from build123d import *

# Parameters (mm, degrees)
SKETCH2_R           = 46.875
BOSS_EXTRUDE1_DEPTH = 3


with BuildPart() as part:
    # Sketch1 → Revolve1 (revolve)
    with BuildSketch(Plane.XY, mode=Mode.PRIVATE) as revolve1_sk:
        Polygon((-48.883652299488276, 0), (-156.25, 61.6327346895418), (-155.75215375739506, 62.5), (-46.875, 0), align=None)
    revolve(revolve1_sk.sketch.rotate(Axis((0, 0, 0), (0, 1, 0)), 90), axis=Axis((0, 0, 0), (0, 1, 0)))



with BuildPart() as body_2:
    # Sketch2 → Boss-Extrude1 (new body)
    with BuildSketch(Plane(origin=(0, 0, 0), x_dir=(1, 0, 0), z_dir=(0, 1, 0))):
        Polygon((-156.24999999999994, -156.25), (156.25000000000003, -156.25), (156.25, 155.75215375739506), (-156.24999999999994, 155.75215375739506), align=None)
        with Locations(Location((8.327e-14, -0.24892312130248007, 0), (0, 0, 270))):
            Circle(SKETCH2_R, mode=Mode.SUBTRACT)
    extrude(amount=-BOSS_EXTRUDE1_DEPTH)


with BuildPart() as part_1:
    add(part.part)

    add(body_2.part)  # Revolve2 merges body 2
    # Sketch3 → Revolve2 (revolve)
    with BuildSketch(Plane.XY, mode=Mode.PRIVATE) as revolve2_sk:
        with BuildLine():
            Line((-65.84427513417332, 9.73610064724726), (-48.88365229948828, 0))
            Line((-48.88365229948828, 0), (-68.44009325263127, 0))
            ThreePointArc((-68.44009325263127, 0), (-63.40199024858691, 3.8708478952321843), (-65.84427513417332, 9.73610064724726))
        make_face()
    revolve(revolve2_sk.sketch.rotate(Axis((0, 0, 0), (0, 1, 0)), 270), axis=Axis((0, 0, 0), (0, 1, 0)))


solid = part_1.part
Check sheet for the modelled part. Datum: model origin and axes. Units: mm. Coordinates: 2 decimals unless noted, no trailing zeros. Loops run counter-clockwise (first coordinate to the right, second up) from the corner with the lowest first, then second, coordinate; pieces in that order, holes last. Notation, with made-up numbers: (2.25, 6) -> (16.25, 6) arc R26 ccw to (16.25, 42) -> close; hole circle Ø9 at (0, 56.25). An arc over 180 degrees is marked (long way). Write item = value, one per line. Start each with the question number.
1. Section check B-B on y = 48. Record the cut outline in (x, z).
2. Draft check along Y on faces 1 (the flat face through (-37, -3, -37)), 2 (the conical face through (-69.799, 12.983, -15.5)), 3 (the conical face through (-50.921, 3.035, -11.308)). Enter one of: released by +Y, released by -Y, zero draft, split by the parting line, or undercut.
3. Section check A-A on x = 0. Record the cut outline in (y, z) (3 decimals), then the cut area to 3 significant figures.
4. Material ranges on line 1 (Y direction, x = 106, z = -136.5); line 2 (X direction, y = 51, z = 21); line 3 (Y direction, x = -6, z = 116), recorded low to high.
5. Depth check by flat-ended pin: P1, Ø2, axis at x = 5, y = 9, coming from the +Z side; P2, Ø5, axis at y = 12, z = -43.5, coming from the -X side; P3, Ø8, axis at y = 23.5, z = -54, coming from the -X side. Enter the tip coordinate at first touch or a pass-through.
Responses:
q1.outline = circle Ø265 at (0, 0); hole circle Ø260.99 at (0, 0)
q2.face_1 = released by -Y
q2.face_2 = undercut
q2.face_3 = released by +Y
q3.outline = (-3, -155.752) -> (0, -155.752) -> (0, -68.44) arc R5.214 cw to (9.736, -65.844) -> (61.633, -156.25) -> (62.5, -155.752) -> (0, -46.875) -> (0, -46.626) -> (-3, -46.626) -> close; (-3, 47.124) -> (0, 47.124) -> (0, 46.875) -> (62.5, 155.752) -> (61.633, 156.25) -> (9.736, 65.844) arc R5.214 cw to (0, 68.44) -> (0, 156.25) -> (-3, 156.25) -> close
q3.area = 1,040 mm2
q4.line_1 = -3 to 0
q4.line_2 = -136.12 to -134.08, 134.08 to 136.12
q4.line_3 = -3 to 0, 38.62 to 39.77
q5.P1 = 66.12
q5.P2 = -60.33
q5.P3 = -80.74
